The drawing under review shows one solid part. Ordinate dimensions are in mm from its lowest x, y, z. A direction names the side the tool comes from. Give positions to 0.01 mm unless a question says otherwise; leave off trailing zeros. Write each loop counter-clockwise with the first axis right and the second up, starting at its lowest first coordinate (ties: lowest second). Pieces come first, ordered by that corner, then holes. Notation, with made-up numbers: (35.5, 23.5) - (93.5, 23.5) arc R13 cw to (93.5, 35.5) - close; hole circle Ø7 at (55, 33). An arc over 180 degrees is marked (long way). Write item = value, one per line.
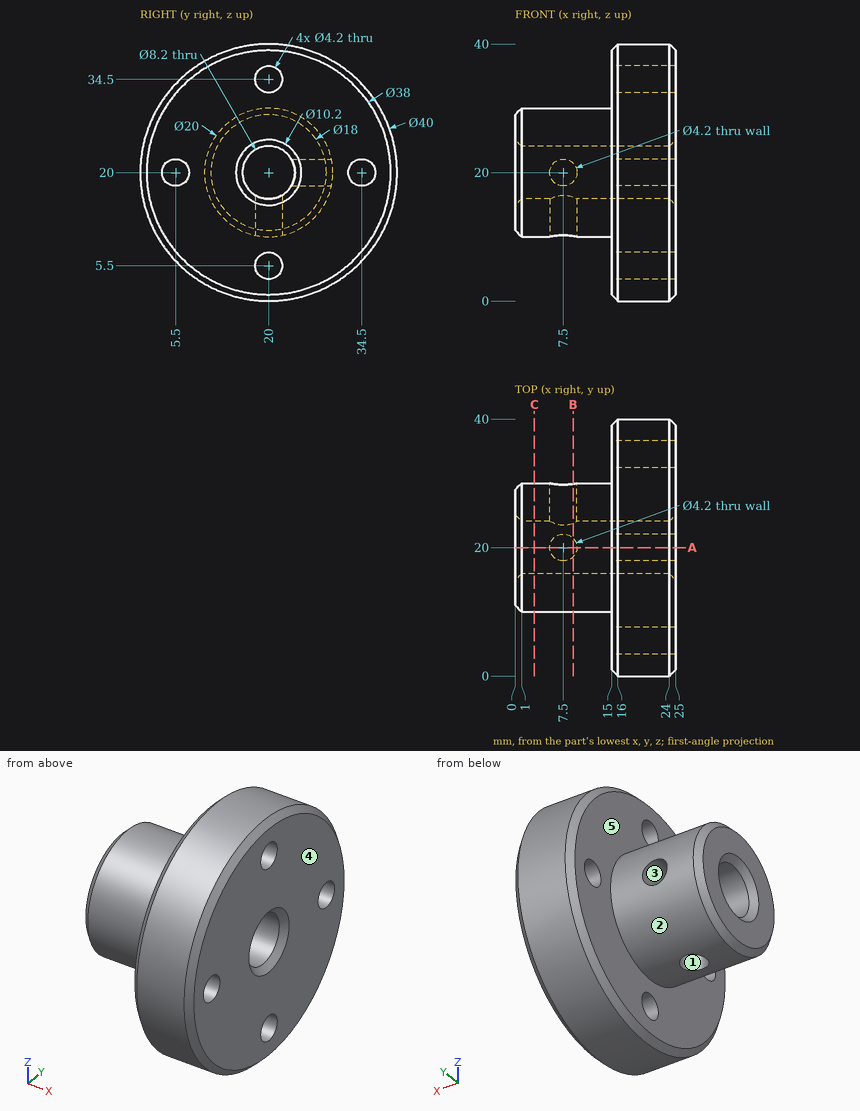
1. Take a section at B-B on x = 9. Give the boundary of the cut face in (y, z), and give its area (3 significant figures).
Findings below:
outline = (18.53, 10.11) - (18.53, 16.17) arc R4.1 cw (long way) to (23.83, 21.47) - (29.89, 21.47) arc R10 ccw (long way) to start; (21.47, 10.11) arc R10 ccw to (29.89, 18.53) - (23.83, 18.53) arc R4.1 cw to (21.47, 16.17) - close
area = 226 mm²
2. Take a section at C-C on x = 3. Give the boundary of the cut face in (y, z), and give its area (3 significant figures).
Findings below:
outline = circle Ø20 at (20, 20); hole circle Ø8.2 at (20, 20)
area = 261 mm²
3. Machinability: for the marked faces 4 and 5, which of the approach directions +Z, -Z, +X, -X, +Y, -Y give a long, thin tool a straight path to every point of the face, cutting with its end or side? Answer none if there is none.
Findings below:
face_4 = +Z, -Z, +X, +Y, -Y
face_5 = -X
4. Insertion check: P1, Ø4, axis at x = 7.5, z = 20, coming from the +Y side; P2, Ø8, axis at x = 13, z = 22.5, coming from the -Y side; P3, Ø8, axis at x = 11.5, z = 29.5, coming from the -Y side; P4, Ø10, axis at x = 3, y = 15.5, coming from the +Z side. Each pin has a flat end and moves straight along its axis. Give the tip position at first contact, or say it passes through.
Findings below:
P1 = 16.42
P2 = 0
P3 = 2.54
P4 = 30
5. Take a section at A-A on y = 20. Count the separate pieces of the cut face and the enclosed holes in it, and give its area (3 significant figures).
Findings below:
separate_pieces = 5
enclosed_holes = 0
area = 381 mm²
6. Draft analysis for pull direction Z (two halves, no side actions). For the marked faces 1, 2 and 3, state which applies: +Z half, -Z half, draft (parallel to the pull), parting line (faces both ways), or undercut.
Findings below:
face_1 = draft
face_2 = parting line
face_3 = undercut
7. For line 1 (X direction, y = 20, z = 13.75); line 2 (Z direction, x = 7.5, y = 28.25); line 3 (X direction, y = 12, z = 7), list the stretches that pass through material, from the lowest coordinate up. Write a range as from..to.
Findings below:
line_1 = 0..5.4, 9.6..25
line_2 = 14.35..17.9, 22.1..25.65
line_3 = 15..25
